from build123d import *

# Parameters (mm, degrees)
SKETCH_W     = 46
SKETCH_H     = 10
SKETCH_R     = 1.2
SKETCH_R_2   = 1.5
PAD_DEPTH    = 10
SKETCH001_R  = 1.2
POCKET_DEPTH = 10.001


with BuildPart() as part:
    # Sketch → Pad (new body)
    with BuildSketch(Plane.XY):
        with Locations((23, 5)):
            Rectangle(SKETCH_W, SKETCH_H)
        with Locations((15, 6)):
            Circle(SKETCH_R, mode=Mode.SUBTRACT)
        with Locations((39, 6)):
            Circle(SKETCH_R, mode=Mode.SUBTRACT)
        with Locations((10, 5)):
            Circle(SKETCH_R_2, mode=Mode.SUBTRACT)
    extrude(amount=PAD_DEPTH)

    # Sketch001 → Pocket (cut, through all)
    with BuildSketch(Plane(origin=(0, 10, 0), x_dir=(-1, 0, 0), z_dir=(0, 1, 0))):
        with Locations((-15, 5)):
            Circle(SKETCH001_R)
        with Locations((-39, 5)):
            Circle(SKETCH001_R)
    extrude(amount=-POCKET_DEPTH, mode=Mode.SUBTRACT)


solid = part.part
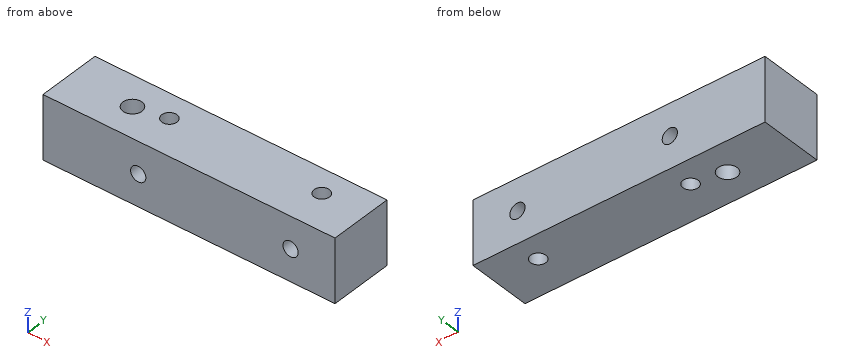
Verification items for the finished model (mm, model axes). Give positions to 0.01 mm unless a question says otherwise; leave off trailing zeros. Loops run counter-clockwise (first coordinate to the right, second up) from the corner with the lowest first, then second, coordinate; pieces in that order, holes last.
1) Sectioned sample at C-C, the plane y = 3. Enter the section's corners in (x, z).
2) Depth check by flat-ended pin: pin 1 Ø1.9 at (x, y) = (39, 6) entering from -Z. Enter the tip coordinate at first touch or a pass-through.
3) Sectioned sample at D-D, the plane x = 10. Enter the section's corners in (y, z), then the cut area to 3 significant figures.
4) Thickness scan on line 1 along X through (y, z) = (0.75, 4.75); line 2 along Z through (x, y) = (15, 4.2); line 3 along X through (y, z) = (6.75, 9). Record the ranges inside material, lowest first.
5) Sectioned sample at A-A, the plane z = 1.5. Enter the section's corners in (x, y), then the cut area to 3 significant figures.
6) Sectioned sample at B-B, the plane x = 39. Enter the section's corners in (y, z).
Answers:
1. outline: (0, 0) - (46, 0) - (46, 10) - (0, 10) - close; hole circle Ø2.4 at (15, 5); hole circle Ø2.4 at (39, 5)
2. pin 1: passes through
3. outline: (0, 0) - (3.5, 0) - (3.5, 10) - (0, 10) - close; (6.5, 0) - (10, 0) - (10, 10) - (6.5, 10) - close
3. area: 70.0 mm2
4. line 1: x = 0 to 13.83, 16.17 to 37.83, 40.17 to 46
4. line 2: z = 0 to 3.8, 6.2 to 10
4. line 3: x = 0 to 14.06, 15.94 to 38.06, 39.94 to 46
5. outline: (0, 0) - (46, 0) - (46, 10) - (0, 10) - close; hole circle Ø3 at (10, 5); hole circle Ø2.4 at (15, 6); hole circle Ø2.4 at (39, 6)
5. area: 444 mm2
6. outline: (0, 0) - (4.8, 0) - (4.8, 3.8) - (0, 3.8) - close; (0, 6.2) - (4.8, 6.2) - (4.8, 10) - (0, 10) - close; (7.2, 0) - (10, 0) - (10, 3.8) - (7.2, 3.8) - close; (7.2, 6.2) - (10, 6.2) - (10, 10) - (7.2, 10) - close
